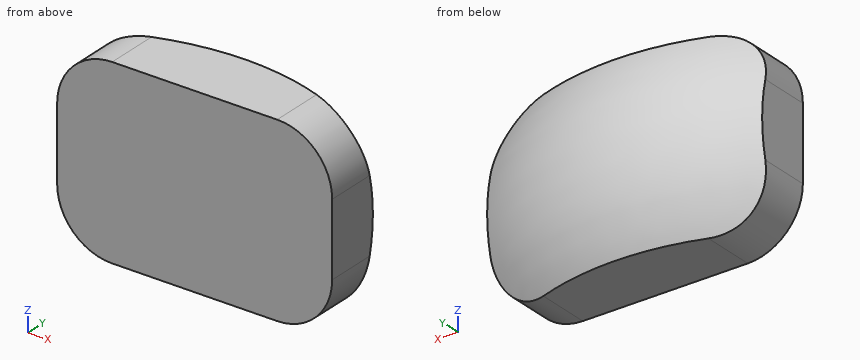
from build123d import *

# Parameters (mm, degrees)
ESQUISSE2_W        = 150
ESQUISSE2_H        = 100
BOSS_EXTRU_1_DEPTH = 50
CONG_1_R           = 30


with BuildPart() as part:
    # Esquisse2 → Boss.-Extru.1 (new body)
    with BuildSketch(Plane(origin=(0, 0, 0), x_dir=(1, 0, 0), z_dir=(0, 1, 0))):
        Rectangle(ESQUISSE2_W, ESQUISSE2_H)
    extrude(amount=BOSS_EXTRU_1_DEPTH)

    # Enlèvement de matière-Balayage1: sweep along a path in Esquisse3
    with BuildLine(Plane.XY) as enl_vement_de_mati_re_balayage1_path:
        ThreePointArc((111.803398875, 0), (0, 50), (-111.803398875, 0))
    # Esquisse4 → Enlèvement de matière-Balayage1 (sweep, cut)
    with BuildSketch(Plane(origin=(0, 0, 0), x_dir=(0, 0, -1), z_dir=(1, 0, 0))):
        with BuildLine():
            Line((-86.602540378, 0), (-86.602540378, 100))
            Line((-86.602540378, 100), (86.602540378, 100))
            Line((86.602540378, 100), (86.602540378, 0))
            ThreePointArc((86.602540378, 0), (0, 50), (-86.602540378, 0))
        make_face()
    sweep(path=enl_vement_de_mati_re_balayage1_path.line, mode=Mode.SUBTRACT)

    # Congé1
    cong_1_edges = [part.edges().sort_by_distance(p)[0] for p in [
        (-75, 7.086018511, 50),
        (-75, 7.086018511, -50),
        (75, 7.086018511, -50),
        (75, 7.086018511, 50),
    ]]
    fillet(cong_1_edges, radius=CONG_1_R)


solid = part.part
Geometry check sheet. Reference: the model listing, model coordinates, mm. Coordinates: 2 decimals unless noted, no trailing zeros. Order: outer loops, then holes, each group sorted by start corner. A loop starts at its lowest first (then second) coordinate and runs counter-clockwise, first axis right, second up. Notation, with made-up numbers: (-14.75, 61) -> (7.25, 61) arc R26 cw to (7.25, 87) -> close; hole circle Ø10 at (72.25, -33.75). An arc over 180 degrees is marked (long way). Use a Markdown table: item, result. Add a question column.
1. Go/stop test with a flat-tipped pin: pin 1 Ø5 at (y, z) = (8.5, -38.5) entering from +X. Record where the tip stops, or that it passes through.
2. Cross-section at A-A (y = 14.5). Enter the section's corners in (x, z), and give its area (3 significant figures).
3. Material ranges on L1, parallel to Y at x = 3.5, z = 31; L2, parallel to X at y = 13, z = 20.5; L3, parallel to Y at x = -9.5, z = 33, recorded low to high.
Filled sheet:
| question | item | result |
|---|---|---|
| 1 | pin 1 | x = 70.38 |
| 2 | outline | (-75, -20) arc R30 ccw to (-45, -50) -> (45, -50) arc R30 ccw to (75, -20) -> (75, 20) arc R30 ccw to (45, 50) -> (-45, 50) arc R30 ccw to (-75, 20) -> close |
| 2 | area | 14,200 mm2 |
| 3 | L1 | 0 to 45.03 |
| 3 | L2 | -75 to 75 |
| 3 | L3 | 0 to 44.09 |
